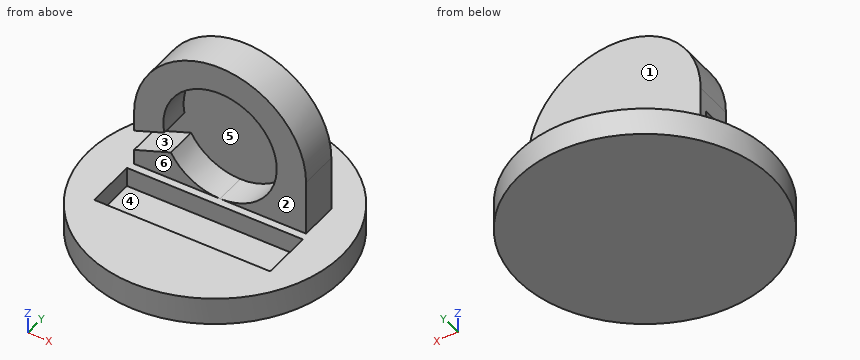
```python
from build123d import *

# Parameters (mm, degrees)
F0_R     = 32.5
F0_W     = 45
F0_H     = 13
F1_DEPTH = 7
F2_DEPTH = 2
F5_DEPTH = 10
F6_START = -8
F6_DEPTH = 2


with BuildPart() as f1:
    # F0 (on Top) → F1 (new body)
    with BuildSketch(Plane.XY):
        Circle(F0_R)
        with Locations((0, -6.5)):
            Rectangle(F0_W, F0_H, mode=Mode.SUBTRACT)
    extrude(amount=F1_DEPTH)

    # F0 (on Top) → F2 (join)
    with BuildSketch(Plane.XY):
        with Locations((0, -6.5)):
            Rectangle(F0_W, F0_H)
    extrude(amount=F2_DEPTH)

    # F4 (on offset) → F5 (join)
    with BuildSketch(Plane.XZ.offset(-2)):
        with BuildLine():
            ThreePointArc((-14.280714402, 18.9670594471), (9.3159717217, 32.6214478116), (-2.92e-08, 7))
            Line((-2.92e-08, 7), (22, 7))
            Line((22, 7), (22, 21.1483523101))
            ThreePointArc((22, 21.1483523101), (0, 43.1483523101), (-22, 21.1483523101))
            Line((-22, 21.1483523101), (-22, 16.1574692596))
            Line((-22, 16.1574692596), (-14.280714402, 18.9670594471))
        make_face()
        with BuildLine():
            ThreePointArc((-2.92e-08, 7), (-7.2603860428, 8.9479555621), (-12.5706136854, 14.2685963432))
            Line((-12.5706136854, 14.2685963432), (-22, 10.8365803972))
            Line((-22, 10.8365803972), (-22, 7))
            Line((-22, 7), (-2.92e-08, 7))
        make_face()
    extrude(amount=-F5_DEPTH)

    # F4 (on offset) → F6 (join)
    with BuildSketch(Plane.XZ.offset(-2).offset(F6_START)):
        with BuildLine():
            Line((-22, 10.8365803972), (-12.5706136854, 14.2685963432))
            ThreePointArc((-12.5706136854, 14.2685963432), (-7.2603860428, 8.9479555621), (-2.92e-08, 7))
            ThreePointArc((-2.92e-08, 7), (9.3159717217, 32.6214478116), (-14.280714402, 18.9670594471))
            Line((-14.280714402, 18.9670594471), (-22, 16.1574692596))
            Line((-22, 16.1574692596), (-22, 10.8365803972))
        make_face()
    extrude(amount=-F6_DEPTH)


solid = f1.part
```
The model under review builds one solid part; all positions refer to its coordinate system, in mm. Face numbers are marked on the shaded views. A direction names the side the tool comes from. Round coordinates to 2 decimals unless told otherwise and drop trailing zeros. Order: outer loops, then holes, each group sorted by start corner. A loop starts at its lowest first (then second) coordinate and runs counter-clockwise, first axis right, second up. Notation, with made-up numbers: (1, 89) -> (13, 89) arc R18 cw to (13, 121) -> close; hole circle Ø5 at (19, 42). An arc over 180 degrees is marked (long way). One line per item, written item: value. Start each with the question number.
Q1. Machinability: for the marked faces 1, 2 and 3, which of the approach directions +Z, -Z, +X, -X, +Y, -Y give a long, thin tool a straight path to every point of the face, cutting with its end or side? Answer none if there is none.
Q2. Take a section at B-B (z = 22.5). Write out the cut boundary in (x, y).
Q3. Wall thickness on line 1 (Z direction, x = 0, y = 7.75); line 2 (Y direction, x = 15.5, z = 27.5); line 3 (Z direction, x = 16.5, y = -18.5): over which ranges is each line inside the solid? List them lowest first.
Q4. Take a section at D-D (z = 8.5). Write out the cut boundary in (x, y), and give its area (3 significant figures).
Q5. Clearance check with flat-ended pins moving along their axes: pin 1 Ø10.5 at (x, y) = (-1.5, -7.5) entering from +Z; pin 2 Ø5.5 at (x, z) = (-1, 5) entering from -Y; pin 3 Ø10 at (x, y) = (-11, 19.5) entering from +Z; pin 4 Ø4 at (x, z) = (24.5, 21) entering from -Y. State where each tip first meets the part, or that it passes through.
Q6. Take a section at A-A (x = -16.5). Write out the cut boundary in (y, z).
Q7. Take a section at C-C (y = 5.5). Write out the cut boundary in (x, z), and give its area (3 significant figures).
Q8. Mouldability with a two-part tool opening along Z and no side actions: class the marked faces 4, 5 and 6 as released by +Z, released by -Z, zero draft, split by the parting line, or undercut.
Reported:
1. face 1: +Z, +X, -X, +Y
1. face 2: +Z, +X, -X, -Y
1. face 3: -X, -Y
2. outline: (-21.96, 2) -> (-14.47, 2) -> (-14.47, 10) -> (14.47, 10) -> (14.47, 2) -> (21.96, 2) -> (21.96, 12) -> (-21.96, 12) -> close
3. line 1: z = 0 to 7, 36.01 to 43.15
3. line 2: y = 2 to 12
3. line 3: z = 0 to 7
4. outline: (-22, 2) -> (-6.42, 2) -> (-6.42, 10) -> (6.42, 10) -> (6.42, 2) -> (22, 2) -> (22, 12) -> (-22, 12) -> close
4. area: 337 mm2
5. pin 1: stops at z = 2
5. pin 2: stops at y = -32.5
5. pin 3: stops at z = 7
5. pin 4: passes through
6. outline: (-28, 0) -> (28, 0) -> (28, 7) -> (12, 7) -> (12, 35.7) -> (2, 35.7) -> (2, 18.16) -> (10, 18.16) -> (10, 12.84) -> (2, 12.84) -> (2, 7) -> (0, 7) -> (0, 2) -> (-13, 2) -> (-13, 7) -> (-28, 7) -> close
7. outline: (-32.03, 0) -> (32.03, 0) -> (32.03, 7) -> (22, 7) -> (22, 21.15) arc R22 ccw to (-22, 21.15) -> (-22, 16.16) -> (-14.28, 18.97) arc R14.5 cw (long way) to (-12.57, 14.27) -> (-22, 10.84) -> (-22, 7) -> (-32.03, 7) -> close
7. area: 1,130 mm2
8. face 4: released by +Z
8. face 5: undercut
8. face 6: zero draft
